Source: three-view drawing plus pictorial views. Frame: mm from the lowest corner of the part. A direction names the side the tool comes from. Coordinates: 2 decimals unless noted, no trailing zeros. Write each loop counter-clockwise with the first axis right and the second up, starting at its lowest first coordinate (ties: lowest second). Pieces come first, ordered by that corner, then holes. Notation, with made-up numbers: (-21, 64.25) - (30, 64.25) arc R18 cw to (30, 99.25) - close; hole circle Ø5 at (-20, 1). An arc over 180 degrees is marked (long way). Put each result on its own line as item: value.
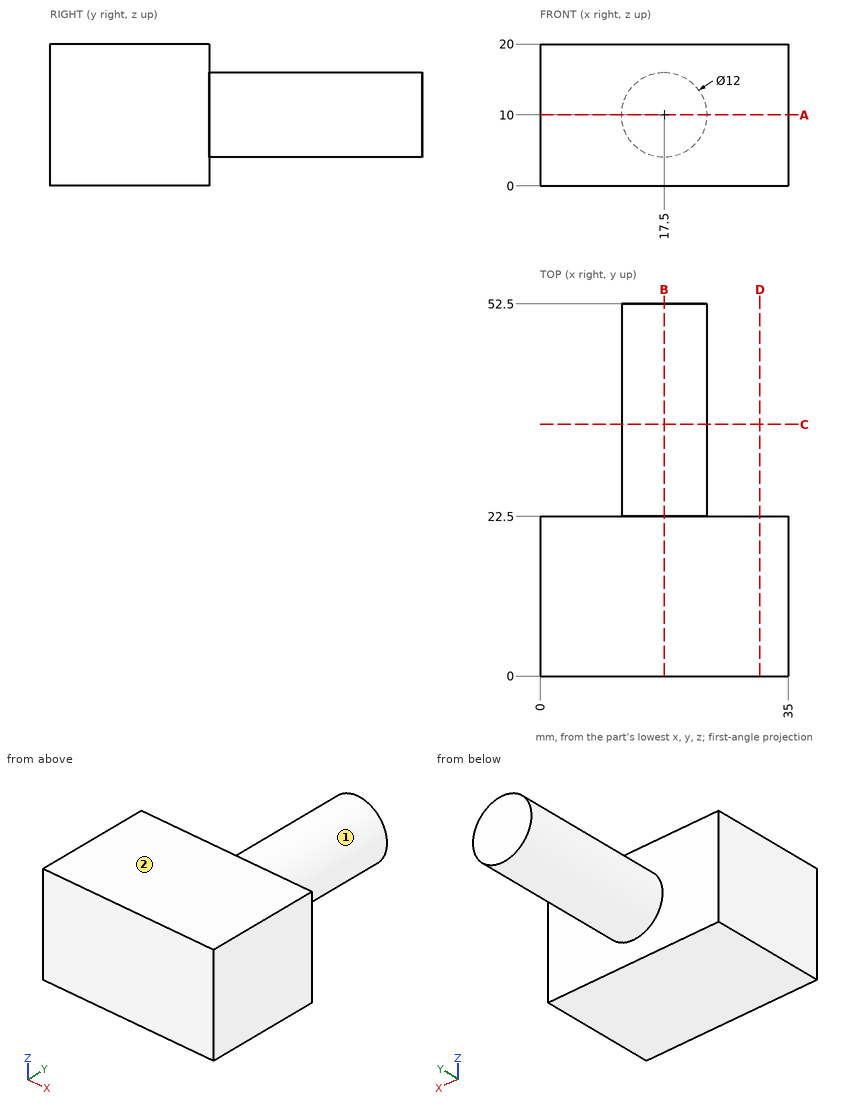
1. Section query C-C (y = 35.5). Return loops of the section in (x, z), then the cut area to 3 significant figures.
Answer below:
outline: circle Ø12 at (17.5, 10)
area: 113 mm²
2. Section query B-B (x = 17.5). Return loops of the section in (y, z), then the cut area to 3 significant figures.
Answer below:
outline: (0, 0) - (22.5, 0) - (22.5, 4) - (52.5, 4) - (52.5, 16) - (22.5, 16) - (22.5, 20) - (0, 20) - close
area: 810 mm²
3. Section query D-D (x = 31). Return loops of the section in (y, z).
Answer below:
outline: (0, 0) - (22.5, 0) - (22.5, 20) - (0, 20) - close
4. Set-up query: the marked faces 1 and 2. Return all of +Z, -Z, +X, -X, +Y, -Y with unobstructed straight access to the full face (end or side cutting, diameter ignored); none if empty.
Answer below:
face 1: +Y
face 2: +Z, +X, -X, +Y, -Y
5. Ray query, probe 1 along Y at (x, z) = (12.5, 4); probe 2 along X at (y, z) = (35, 10); probe 3 along Z at (x, y) = (15, 28.5). Return the intervals inside material, ascending. Write a range as from..to.
Answer below:
probe 1: y = 0..22.5
probe 2: x = 11.5..23.5
probe 3: z = 4.55..15.45
6. Section query A-A (z = 10). Return loops of the section in (x, y).
Answer below:
outline: (0, 0) - (35, 0) - (35, 22.5) - (23.5, 22.5) - (23.5, 52.5) - (11.5, 52.5) - (11.5, 22.5) - (0, 22.5) - close
7. Pin query (flat end, axial travel): pin 1 Ø6 at (y, z) = (34.5, 11.5) entering from +X; pin 2 Ø12 at (x, y) = (29, 41.5) entering from -Z; pin 3 Ø1 at (y, z) = (37.5, 11.5) entering from -X. Return the tip coordinate at first contact, or that it passes through.
Answer below:
pin 1: stops at x = 23.5
pin 2: stops at z = 7.6
pin 3: stops at x = 11.58
